from build123d import *

# Parameters (mm, degrees)
ESQUISSE1_W                      = 25
ESQUISSE1_H                      = 15
BOSS_EXTRU_1_DEPTH               = 39
BOSS_EXTRU_1_2_DEPTH             = 39
ESQUISSE3_W                      = 160
ESQUISSE3_H                      = 15
BOSS_EXTRU_2_DEPTH               = 15
ESQUISSE4_R                      = 5
ESQUISSE4_R_2                    = 4
BOSS_EXTRU_5_DEPTH               = 0.8
ESQUISSE4_6_R                    = 4
BOSS_EXTRU_6_DEPTH               = 7.4
CONG_1_R                         = 10
ESQUISSE5_W                      = 11
ESQUISSE5_H                      = 34
ENL_V_MAT_EXTRU_1_DEPTH          = 97.874970968
CONG_2_R                         = 10
ESQUISSE6_R                      = 1.75
ENL_V_MAT_EXTRU_2_DEPTH          = 101.478903258
ESQUISSE11_R                     = 1.75
TROUS_VIS_SUPPORT_CAPTEURS_DEPTH = 97.000052083
ESQUISSE12_W                     = 33.4
ESQUISSE12_H                     = 4.7
ENCOCHE_CARTE_CAPTEUR_DEPTH      = 97.000052083


with BuildPart() as part:
    # Esquisse1 → Boss.-Extru.1 (new body)
    with BuildSketch(Plane(origin=(0, 0, 0), x_dir=(0, 1, 0), z_dir=(0, 0, 1))):
        with Locations((-45, 0)):
            Rectangle(ESQUISSE1_W, ESQUISSE1_H)
    extrude(amount=BOSS_EXTRU_1_DEPTH)



with BuildPart() as body_2:
    # Esquisse1 → Boss.-Extru.1 2 (new body)
    with BuildSketch(Plane(origin=(0, 0, 0), x_dir=(0, 1, 0), z_dir=(0, 0, 1))):
        with Locations((45, 0)):
            Rectangle(ESQUISSE1_W, ESQUISSE1_H)
    extrude(amount=BOSS_EXTRU_1_2_DEPTH)


with BuildPart() as part_1:
    add(part.part)

    add(body_2.part)  # Boss.-Extru.2 merges body 2
    # Esquisse3 → Boss.-Extru.2 (add)
    with BuildSketch(Plane(origin=(0, 0, 0), x_dir=(0, 1, 0), z_dir=(0, 0, 1))):
        Rectangle(ESQUISSE3_W, ESQUISSE3_H)
    extrude(amount=-BOSS_EXTRU_2_DEPTH)

    # Esquisse4 → Boss.-Extru.5 (add)
    with BuildSketch(Plane(origin=(0, -80, 0), x_dir=(-1, 0, 0), z_dir=(0, -1, 0))):
        with Locations(Location((0, 7.5, 0), (0, 0, 90))):
            Circle(ESQUISSE4_R)
        with Locations(Location((0, 7.5, 0), (0, 0, 90))):
            Circle(ESQUISSE4_R_2, mode=Mode.SUBTRACT)
    boss_extru_5 = extrude(amount=BOSS_EXTRU_5_DEPTH)

    # Esquisse4<6> → Boss.-Extru.6 (add)
    with BuildSketch(Plane(origin=(0, -80, 0), x_dir=(-1, 0, 0), z_dir=(0, -1, 0))):
        with Locations(Location((0, 7.5, 0), (0, 0, 90))):
            Circle(ESQUISSE4_6_R)
    boss_extru_6 = extrude(amount=BOSS_EXTRU_6_DEPTH)

    # Symétrie2: Boss.-Extru.5, Boss.-Extru.6 across plane
    add(boss_extru_5.mirror(Plane.ZX))
    add(boss_extru_6.mirror(Plane.ZX))

    # Congé1
    cong_1_edges = [part_1.edges().sort_by_distance(p)[0] for p in [
        (0, 57.5, 0),
        (0, 32.5, 0),
        (0, -57.5, 0),
        (0, -32.5, 0),
    ]]
    fillet(cong_1_edges, radius=CONG_1_R)

    # Esquisse5 → Enlèv. mat.-Extru.1 (cut, through all)
    with BuildSketch(Plane(origin=(-7.5, 0, 0), x_dir=(0, -1, 0), z_dir=(-1, 0, 0))):
        with Locations((45, 17)):
            Rectangle(ESQUISSE5_W, ESQUISSE5_H)
        with Locations((-45, 17)):
            Rectangle(ESQUISSE5_W, ESQUISSE5_H)
    extrude(amount=-ENL_V_MAT_EXTRU_1_DEPTH, mode=Mode.SUBTRACT)

    # Congé2
    # the kernel refuses this fillet: 10 mm, written as the material it adds along each edge
    with BuildSketch(Plane(origin=(-7.5, 39.5, 0), x_dir=(0, 0, 1), z_dir=(1, 0, 0)), Plane(origin=(-7.5, -39.5, 0), x_dir=(0, -1, 0), z_dir=(1, 0, 0)), Plane(origin=(-7.5, -50.5, 0), x_dir=(0, 0, 1), z_dir=(1, 0, 0))) as cong_2_piece_1:
        with BuildLine():
            CenterArc((CONG_2_R, -CONG_2_R), CONG_2_R, 90, 90)
            Line((0, -CONG_2_R), (0, 0))
            Line((0, 0), (CONG_2_R, 0))
        make_face()
    extrude(amount=15)
    with BuildSketch(Plane(origin=(-7.5, 50.5, 0), x_dir=(0, 0, 1), z_dir=(1, 0, 0))) as cong_2_piece_2:
        with BuildLine():
            CenterArc((CONG_2_R, CONG_2_R), CONG_2_R, 180, 90)
            Line((0, CONG_2_R), (0, 0))
            Line((0, 0), (CONG_2_R, 0))
        make_face()
    extrude(amount=15)

    # Esquisse6 → Enlèv. mat.-Extru.2 (cut, through all)
    with BuildSketch(Plane(origin=(0, 0, 34), x_dir=(1, 0, 0), z_dir=(0, 0, -1))):
        with Locations(Location((0, 45, 0), (0, 0, 180))):
            Circle(ESQUISSE6_R)
        with Locations((0, -45)):
            Circle(ESQUISSE6_R)
    extrude(amount=-ENL_V_MAT_EXTRU_2_DEPTH, mode=Mode.SUBTRACT)

    # Esquisse11 → Trous vis support capteurs (cut, through all)
    with BuildSketch(Plane(origin=(0, 0, 0), x_dir=(0, 1, 0), z_dir=(0, 0, 1))):
        with Locations(Location((20, 0, 0), (0, 0, 270))):
            Circle(ESQUISSE11_R)
        with Locations(Location((-20, 0, 0), (0, 0, 270))):
            Circle(ESQUISSE11_R)
    extrude(amount=-TROUS_VIS_SUPPORT_CAPTEURS_DEPTH, mode=Mode.SUBTRACT)

    # Esquisse12 → Encoche carte capteur (cut, through all)
    with BuildSketch(Plane(origin=(0, 0, 0), x_dir=(0, 1, 0), z_dir=(0, 0, 1))):
        with Locations((-11.675958981, -8.388484641)):
            Rectangle(ESQUISSE12_W, ESQUISSE12_H)
    extrude(amount=-ENCOCHE_CARTE_CAPTEUR_DEPTH, mode=Mode.SUBTRACT)


solid = part_1.part
Read the model definition and answer for the solid it produces. Units are mm, in the model's axes. A direction names the side the tool comes from. Coordinates: 2 decimals unless noted, no trailing zeros. Order: outer loops, then holes, each group sorted by start corner. A loop starts at its lowest first (then second) coordinate and runs counter-clockwise, first axis right, second up. Notation, with made-up numbers: (-40, -32.75) -> (9, -32.75) arc R23 cw to (9, -8.75) -> close; hole circle Ø4 at (14.25, -8.5). An arc over 180 degrees is marked (long way). Answer as a JSON object with one key per item and string values.
1) Consider line 1 along Y through (x, z) = (0, -6.5); line 2 along Y through (x, z) = (6.5, 20); line 3 along X through (y, z) = (45, 35.1). Determine where each line is inside the solid, lowest interval first. Write a range as from..to.
Model answer:
{"line 1": "y = -87.4..-21.75, -18.25..18.25, 21.75..87.4", "line 2": "y = -57.5..-50.5, -39.5..-32.5, 32.5..39.5, 50.5..57.5", "line 3": "x = -7.5..-1.75, 1.75..7.5"}
2) A cutting plane is placed at A-A, the plane z = 35.5. Determine the outline of the cut face in (x, y).
Model answer:
{"outline": "(-7.5, -57.5) -> (7.5, -57.5) -> (7.5, -32.5) -> (-7.5, -32.5) -> close; (-7.5, 32.5) -> (7.5, 32.5) -> (7.5, 57.5) -> (-7.5, 57.5) -> close; hole circle Ø3.5 at (0, -45); hole circle Ø3.5 at (0, 45)"}
3) The mould has two halves that part along X. Classify faces 4 (the face through (0, -32.5, 24)), 5 (the face through (-0.228, -18.265, -7.395)), 6 (the face through (-2.4, 84.1, -4.3)): released by +X, released by -X, zero draft, split by the parting line, or undercut.
Model answer:
{"face 4": "zero draft", "face 5": "undercut", "face 6": "split by the parting line"}
4) Each of these flat-tipped pins is pushed along its axis until it touches: pin 1 (5 mm diameter, centred on x = 4, y = -68.5, fed in from +Z); pin 2 (1 mm diameter, centred on x = -0.5, y = -45.5, fed in from +Z); pin 3 (7.5 mm diameter, centred on x = 2, z = 24.5, fed in from +Y). Where does it stop, or does it pass through?
Model answer:
{"pin 1": "stops at z = 0.11", "pin 2": "stops at z = 1.65", "pin 3": "stops at y = 57.5"}
5) A cutting plane is placed at D-D, the plane x = 0. State how many separate pieces and enclosed holes the cut face has, plus the area to 3 significant figures.
Model answer:
{"separate pieces": "3", "enclosed holes": "0", "area": "3,750 mm²"}
6) A tool of negligible diameter and unlimited length cuts with its end or side. For faces 1 (the face through (0, 57.5, 24)), 2 (the face through (-0.38, 46.71, 36.47)), 3 (the face through (-0.11, -29.49, 2.85)), from which of +Z, -Z, +X, -X, +Y, -Y can it reach the whole face along a straight path? Write none if from no direction.
Model answer:
{"face 1": "+Z, +X, -X, +Y", "face 2": "+Z", "face 3": "+Z, +X, -X"}
7) A cutting plane is placed at C-C, the plane z = 15. Determine the outline of the cut face in (x, y), plus the area to 3 significant figures.
Model answer:
{"outline": "(-7.5, -57.5) -> (7.5, -57.5) -> (7.5, -50.5) -> (-7.5, -50.5) -> close; (-7.5, -39.5) -> (7.5, -39.5) -> (7.5, -32.5) -> (-7.5, -32.5) -> close; (-7.5, 32.5) -> (7.5, 32.5) -> (7.5, 39.5) -> (-7.5, 39.5) -> close; (-7.5, 50.5) -> (7.5, 50.5) -> (7.5, 57.5) -> (-7.5, 57.5) -> close", "area": "420 mm²"}
8) A cutting plane is placed at B-B, the plane y = -20. Determine the outline of the cut face in (x, z).
Model answer:
{"outline": "(-7.5, -15) -> (-1.75, -15) -> (-1.75, 0) -> (-7.5, 0) -> close; (1.75, -15) -> (6.04, -15) -> (6.04, 0) -> (1.75, 0) -> close"}
